Work out the finished part from the listing and answer in its coordinate system (mm). A direction names the side the tool comes from. Give positions to 0.01 mm unless a question says otherwise; leave off trailing zeros. Order: outer loops, then holes, each group sorted by start corner. A loop starts at its lowest first (then second) coordinate and runs counter-clockwise, first axis right, second up. Notation, with made-up numbers: (-15, 63) - (12, 63) arc R10 ccw to (12, 69) - close; hole circle Ø11 at (-22, 48). An arc over 180 degrees is marked (long way). Put each result on its own line as item: value.
```python
from build123d import *

# Parameters (mm, degrees)
SKETCH1_W           = 10
SKETCH1_H           = 5
SKETCH1_R           = 1.6
BOSS_EXTRUDE2_DEPTH = 2
SKETCH2_W           = 1.5
SKETCH2_H           = 5
BOSS_EXTRUDE3_DEPTH = 15
SKETCH3_W           = 8
SKETCH3_H           = 5
SKETCH3_R           = 1.6
BOSS_EXTRUDE4_DEPTH = 2
BOSS_EXTRUDE5_DEPTH = 5


with BuildPart() as part:
    # Sketch1 → Boss-Extrude2 (new body)
    with BuildSketch(Plane(origin=(0, 0, 0), x_dir=(1, 0, 0), z_dir=(0, 1, 0))):
        with Locations((-2, 0.5)):
            Rectangle(SKETCH1_W, SKETCH1_H)
        with Locations((-1, 0.5)):
            Circle(SKETCH1_R, mode=Mode.SUBTRACT)
    extrude(amount=BOSS_EXTRUDE2_DEPTH)

    # Sketch2 → Boss-Extrude3 (add)
    with BuildSketch(Plane.XZ):
        with Locations((-5.75, -0.5)):
            Rectangle(SKETCH2_W, SKETCH2_H)
    extrude(amount=BOSS_EXTRUDE3_DEPTH)

    # Sketch3 → Boss-Extrude4 (add)
    with BuildSketch(Plane.XZ.offset(15)):
        with Locations((-9, -0.5)):
            Rectangle(SKETCH3_W, SKETCH3_H)
        with Locations((-9.5, -0.5)):
            Circle(SKETCH3_R, mode=Mode.SUBTRACT)
    extrude(amount=BOSS_EXTRUDE4_DEPTH)

    # Sketch4 → Boss-Extrude5 (add)
    with BuildSketch(Plane.XY.offset(2)):
        Polygon((4.737702607, -17), (4.737702607, 2), (3, 2), (3, -15), (-5, -15), (-5, -17), align=None)
    extrude(amount=-BOSS_EXTRUDE5_DEPTH)


solid = part.part
```
(1) Section C-C, the plane z = -1.65 is taken. Write down the section's boundary in (x, y).
Geometry check:
outline: (-13, -17) - (-10.61, -17) - (-10.61, -15) - (-13, -15) - close; (-8.39, -17) - (4.74, -17) - (4.74, 2) - (0.11, 2) - (0.11, 0) - (3, 0) - (3, -15) - (-5, -15) - (-5, 0) - (-2.11, 0) - (-2.11, 2) - (-7, 2) - (-7, 0) - (-6.5, 0) - (-6.5, -15) - (-8.39, -15) - close
(2) Given pin 1 (1.5 mm diameter, centred on y = -4, z = -1, fed in from -X); pin 2 (10 mm diameter, centred on x = -10, y = -6.5, fed in from -Z); pin 3 (0.6 mm diameter, centred on y = 1, z = 0, fed in from -X); pin 4 (3 mm diameter, centred on x = -9.5, z = -0.5, fed in from +Y), each flat-ended and moving along its own axis, determine where each tip first touches the part or whether it passes through.
Geometry check:
pin 1: stops at x = -6.5
pin 2: stops at z = -3
pin 3: stops at x = -7
pin 4: passes through
(3) Section D-D, the plane x = -1 is taken. Write down the section's boundary in (y, z), then the cut area to 3 significant figures.
Geometry check:
outline: (-17, -3) - (-15, -3) - (-15, 2) - (-17, 2) - close; (0, -3) - (2, -3) - (2, -2.1) - (0, -2.1) - close; (0, 1.1) - (2, 1.1) - (2, 2) - (0, 2) - close
area: 13.6 mm²
(4) Straight lines are drawn through the part: line 1 (X direction, y = -1, z = 0.5); line 2 (X direction, y = 1.25, z = -0.5); line 3 (Z direction, x = -1, y = 0.7). For each, find the intervals that lie inside material, in ascending order.
Geometry check:
line 1: x = -6.5 to -5, 3 to 4.74
line 2: x = -7 to -2.6, 0.6 to 4.74
line 3: z = -3 to -2.1, 1.1 to 2
(5) Section B-B, the plane x = -9.5 is taken. Write down the section's boundary in (y, z).
Geometry check:
outline: (-17, -3) - (-15, -3) - (-15, -2.1) - (-17, -2.1) - close; (-17, 1.1) - (-15, 1.1) - (-15, 2) - (-17, 2) - close
(6) Section A-A, the plane y = -8 is taken. Write down the section's boundary in (x, z).
Geometry check:
outline: (-6.5, -3) - (-5, -3) - (-5, 2) - (-6.5, 2) - close; (3, -3) - (4.74, -3) - (4.74, 2) - (3, 2) - close
(7) Determine the mould class of faces 1 (the face through (-7, 1, 0)), 2 (the face through (4.738, -8, 0)), 3 (the face through (-4, -17, 0)), 4 (the face through (3, -7, 0)) for opening direction X: pulls with the +X half, pulls with the -X half, needs draft (parallel to the pull), parting line crosses it, or undercut.
Geometry check:
face 1: pulls with the -X half
face 2: pulls with the +X half
face 3: needs draft
face 4: undercut
(8) A tool of negligible diameter and unlimited length cuts with its end or side. For faces 5 (the face through (1, 0, -1)), 6 (the face through (-6.5, -7, -1)), 7 (the face through (-5.5, -8.2, -3)), 8 (the face through (-5.5, -8.2, 2)), 9 (the face through (0.48, 0.99, 0.11)), from which of +Z, -Z, +X, -X, +Y, -Y can it reach the whole face along a straight path? Write none if from no direction.
Geometry check:
face 5: +Z, -Z
face 6: +Z, -Z, -X
face 7: -Z, +X, -X, +Y, -Y
face 8: +Z, +X, -X, +Y, -Y
face 9: +Y
